CAD build for the part. Positions are in the model's coordinates, mm. A direction names the side the tool comes from. Round coordinates to 2 decimals unless told otherwise and drop trailing zeros. Write each loop counter-clockwise with the first axis right and the second up, starting at its lowest first coordinate (ties: lowest second). Pieces come first, ordered by that corner, then holes. Notation, with made-up numbers: M 57.25,66.5 L 72.25,66.5 A25 cw 72.25,105.5 Z; hole C -20,48.5 d1. An arc over 180 degrees is marked long. Write each question's results on one line, items separated by ' | '. Start each with the question number.
Autodesk Inventor part; units mm, degrees
ref_plane "YZ Plane" through (0, 0, 0) normal (1, 0, 0) x (0, 1, 0)
ref_plane "XZ Plane" through (0, 0, 0) normal (0, 1, 0) x (-1, 0, 0)
ref_plane "XY Plane" through (0, 0, 0) normal (0, 0, 1) x (1, 0, 0)
sketch "Szkic1" plane through (0, 0, 0) normal (0, 1, 0) x (-1, 0, 0)
  line L0 (0, 0) -> (-50, 0)
  line L1 (-50, 0) -> (-50, -50)
  line L2 (-50, -50) -> (0, -50)
  line L3 (0, -50) -> (0, 0)
  line L4 (-2, -2) -> (-48, -2)
  line L5 (-48, -2) -> (-48, -48)
  line L6 (-48, -48) -> (-2, -48)
  line L7 (-2, -48) -> (-2, -2)
  dimension "d0" = 50
  dimension "d1" = 50
  dimension "d2" = 2
extrude "Wyciągnięcie proste1" add sketch "Szkic1" along normal blind 2
sketch "Szkic2" plane through (0, 2, 0) normal (0, 1, 0) x (1, 0, 0)
  line L0 (50, 0) -> (50, 50)
  line L1 (50, 50) -> (0, 50)
  line L2 (0, 50) -> (0, 0)
  line L3 (0, 0) -> (50, 0)
  line L4 (2, 2) -> (2, 48)
  line L5 (2, 48) -> (48, 48)
  line L6 (48, 48) -> (48, 2)
  line L7 (48, 2) -> (2, 2)
  line L8 (0, 50) -> (0, 0)
  line L9 (0, 0) -> (2, 0)
  line L10 (2, 0) -> (2, 2)
  line L11 (2, 2) -> (0, 2)
  line L12 (0, 2) -> (0, 0)
  line L13 (2, 48) -> (0, 48)
  line L14 (0, 48) -> (0, 50)
  line L15 (0, 50) -> (2, 50)
  line L16 (2, 50) -> (2, 48)
  line L17 (0, 0) -> (50, 0)
  line L18 (50, 0) -> (48, 0)
  line L19 (48, 0) -> (48, 2)
  line L20 (48, 2) -> (50, 2)
  line L21 (50, 2) -> (50, 0)
  line L22 (2, 48) -> (48, 48)
  line L23 (48, 48) -> (50, 48)
  line L24 (50, 48) -> (50, 50)
  line L25 (50, 50) -> (48, 50)
  line L26 (48, 50) -> (48, 48)
extrude "Wyciągnięcie proste2" add sketch "Szkic2" along normal blind 46 contours L3 L19 L20 L0 | L23 L26 L1 L0 | L3 L2 L11 L10 | L13 L2 L1 L16
sketch "Szkic3" plane through (0, 48, 0) normal (0, 1, 0) x (1, 0, 0)
  line L0 (48, 50) -> (2, 50)
  line L1 (50, 0) -> (50, 50)
  line L2 (0, 0) -> (50, 0)
  line L3 (0, 50) -> (0, 0)
  line L4 (50, 50) -> (0, 50)
  line L5 (2, 2) -> (2, 48)
  line L6 (48, 2) -> (2, 2)
  line L7 (48, 48) -> (48, 2)
  line L8 (2, 48) -> (48, 48)
extrude "Wyciągnięcie proste3" add sketch "Szkic3" along normal blind 2
properties part number "wymiar"
1) 3-axis set-ups, long thin cutter, end or side, ignore diameter. For faces 1 (the face through (23, 49, 0)), 2 (the face through (49, 48, -25)), 3 (the face through (2, 25, -1)), 4 (the face through (25, 1, -2)): which of +Z, -Z, +X, -X, +Y, -Y reach the whole face in a straight line?
2) Pull direction Z, two halves, no side cores. Call faces 5 (the face through (27, 49, -50)), 6 (the face through (25, 49, -2)), 7 (the face through (0, 49, -27)): pulls with the +Z half, pulls with the -Z half, needs draft (parallel to the pull), parting line crosses it, or undercut.
3) Saw through at A-A, the plane y = 36. Write the cut outline in (x, z).
Filled sheet:
1) face 1: +Z, +X, -X, +Y, -Y | face 2: +X, -X | face 3: +Z, -Z | face 4: +Y, -Y
2) face 5: pulls with the -Z half | face 6: undercut | face 7: needs draft
3) outline: M 0,-50 L 2,-50 L 2,-48 L 0,-48 Z; M 0,-2 L 2,-2 L 2,0 L 0,0 Z; M 48,-50 L 50,-50 L 50,-48 L 48,-48 Z; M 48,-2 L 50,-2 L 50,0 L 48,0 Z
